Input: part model. Units: mm. Frame: model coordinates. Give positions to 0.01 mm unless a question says otherwise; leave off trailing zeros. Loops run counter-clockwise (first coordinate to the right, second up) from the corner with the lowest first, then second, coordinate; pieces in that order, holes last. Notation, with made-up numbers: M -13,23 L 7,23 A17 cw 7,34 Z; hole C 34,-31.75 d4. An arc over 180 degrees is marked long. Answer as a JSON object with one key per item and string values. Group by question number.
1) Ray query, L1, parallel to Y at x = 49, z = 0.7; L2, parallel to X at y = 41.5, z = 1.35. Return the intervals inside material, ascending.
2) Section query A-A on x = 58. Return loops of the section in (y, z).
3) First-contact query: P1, Ø0.9, axis at y = 44, z = 1.5, coming from the +X side. Flat tip, straight axial feed; report the tip coordinate or a pass-through.
4) Section query C-C on y = 34.5. Return loops of the section in (x, z), plus the area to 3 significant figures.
5) Section query B-B on z = 1.05. Return loops of the section in (x, y).
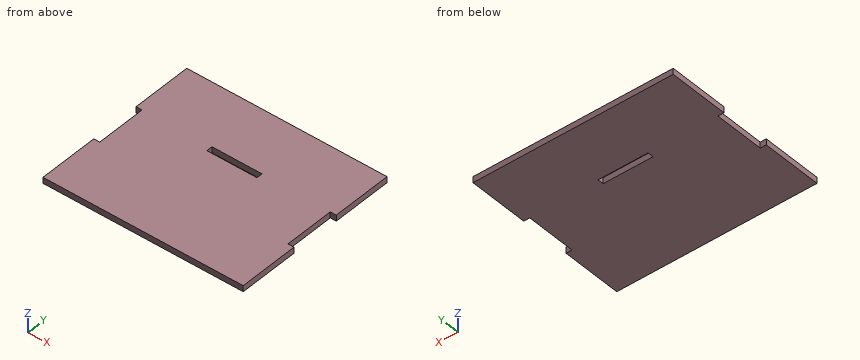
Autodesk Inventor part; units mm, degrees
ref_plane "YZ Plane" through (0, 0, 0) normal (1, 0, 0) x (0, 1, 0)
ref_plane "XZ Plane" through (0, 0, 0) normal (0, 1, 0) x (-1, 0, 0)
ref_plane "XY Plane" through (0, 0, 0) normal (0, 0, 1) x (1, 0, 0)
sketch "Sketch1" plane through (0, 0, 0) normal (0, 0, 1) x (1, 0, 0)
  line L0 (0, 0) -> (100, 0)
  line L1 (100, 0) -> (100, 30)
  line L2 (100, 30) -> (97, 30)
  line L3 (97, 30) -> (97, 55)
  line L4 (97, 55) -> (100, 55)
  line L5 (100, 55) -> (100, 85)
  line L6 (100, 85) -> (0, 85)
  line L7 (0, 85) -> (0, 55)
  line L8 (0, 55) -> (3, 55)
  line L9 (3, 55) -> (3, 30)
  line L10 (3, 30) -> (0, 30)
  line L11 (0, 30) -> (0, 0)
  line L12 (50, 0) -> (50, 52.5) construction
  line L13 (50, 52.5) -> (50, 80) construction
  circle A0 centre (50, 80) radius 27.5 construction
  line L14 (50, 80) -> (50, 85) construction
  line L15 (50, 107.5) -> (50, 85) construction
  line L16 (50, 52.5) -> (50, 60.5) construction
  line L17 (50, 60.5) -> (50, 70.5) construction
  line L18 (50, 52.5) -> (50, 55.5) construction
  line L19 (50, 55.5) -> (50, 52.5) construction
  line L20 (50, 55.5) -> (62.5, 55.5)
  line L21 (62.5, 55.5) -> (62.5, 52.5)
  line L22 (62.5, 52.5) -> (37.5, 52.5)
  line L23 (37.5, 52.5) -> (37.5, 55.5)
  line L24 (37.5, 55.5) -> (50, 55.5)
  dimension "d15" = 55
  dimension "d0" = 100
  dimension "d1" = 30
  dimension "d3" = 25
  dimension "d4" = 3
  dimension "d5" = 30
  dimension "d6" = 100
  dimension "d7" = 30
  dimension "d8" = 3
  dimension "d9" = 25
  dimension "d10" = 3
  dimension "d13" = 52.5
  dimension "d14" = 27.5
  dimension "d17" = 8
  dimension "d18" = 10
  dimension "d21" = 3
  dimension "d22" = 12.5
  dimension "d23" = 3
  dimension "d24" = 25
  dimension "d25" = 3
  dimension "d26" = 52.5
extrude "Extrusion1" add sketch "Sketch1" along normal blind 3
properties part number "Samping"
Output:
{
 "1": {"L1": "y = 0 to 52.5, 55.5 to 85", "L2": "x = 3 to 97"},
 "2": {"outline": "M 0,0 L 52.5,0 L 52.5,3 L 0,3 Z; M 55.5,0 L 85,0 L 85,3 L 55.5,3 Z"},
 "3": {"P1": "stops at x = 97"},
 "4": {"outline": "M 3,0 L 97,0 L 97,3 L 3,3 Z", "area": "282 mm^2"},
 "5": {"outline": "M 0,0 L 100,0 L 100,30 L 97,30 L 97,55 L 100,55 L 100,85 L 0,85 L 0,55 L 3,55 L 3,30 L 0,30 Z; hole M 37.5,52.5 L 62.5,52.5 L 62.5,55.5 L 37.5,55.5 Z"}
}
